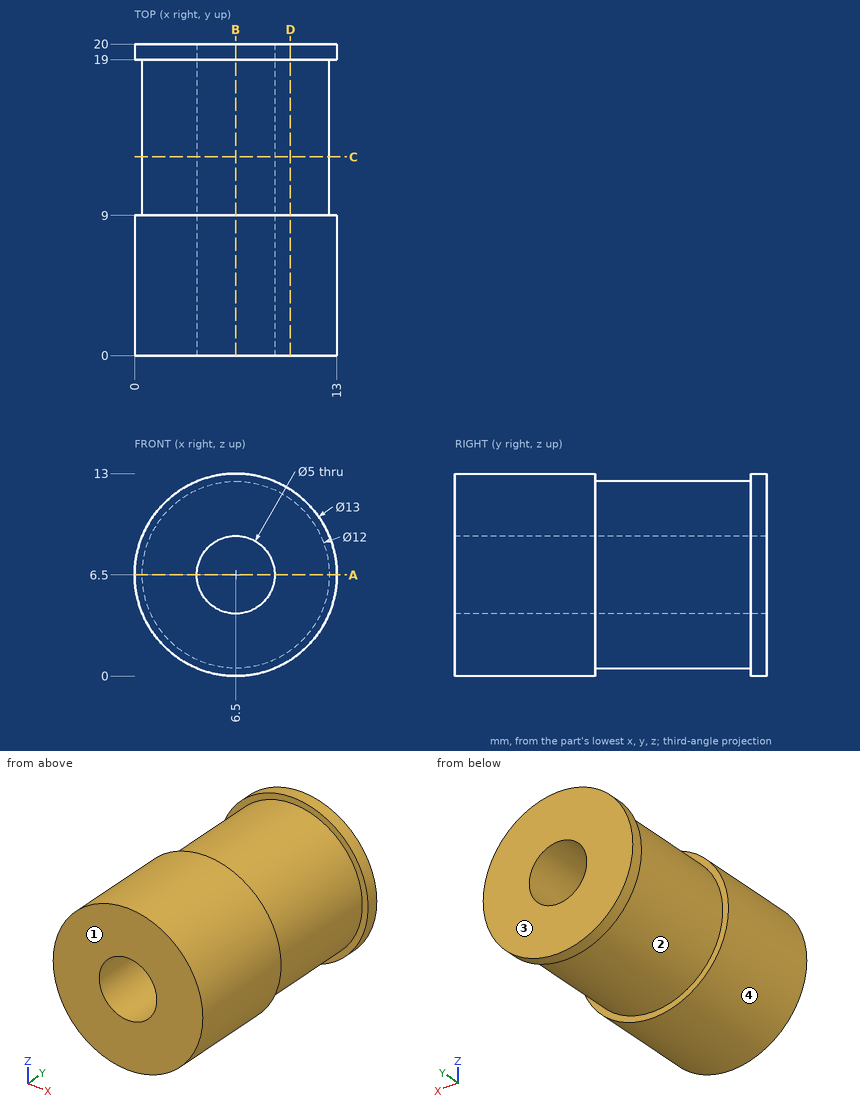
Here's the drawing with two shaded views (mm, measured from the low corner). I have some questions. Round coordinates to 2 decimals unless told otherwise and drop trailing zeros. Order: outer loops, then holes, each group sorted by start corner. A loop starts at its lowest first (then second) coordinate and runs counter-clockwise, first axis right, second up. Notation, with made-up numbers: M 22.5,-22.5 L 81.5,-22.5 A29 ccw 81.5,15.5 Z; hole C 19.25,51 d7. An arc over 180 degrees is marked long. Answer in a Markdown table with one row per item.
Item 1: Imagine slicing it at D-D, the plane x = 10. Write out the boundary of the cut face in (y, z).
A:
| item | result |
|---|---|
| outline | M 0,1.02 L 9,1.02 L 9,1.63 L 19,1.63 L 19,1.02 L 20,1.02 L 20,11.98 L 19,11.98 L 19,11.37 L 9,11.37 L 9,11.98 L 0,11.98 Z |
Item 2: Thinking about a two-plate mould opening in Y: for the marked faces 1, 2, 3 and 4, which applies, +Y half, -Y half, draft (parallel to the pull), parting line (faces both ways), or undercut?
A:
| item | result |
|---|---|
| face 1 | -Y half |
| face 2 | undercut |
| face 3 | +Y half |
| face 4 | draft |
Item 3: I'm going to push flat-ended pins straight in: pin 1 (5 mm diameter, centred on x = 10, y = 18, fed in from -Z); pin 2 (2 mm diameter, centred on y = 7, z = 10.5, fed in from -X); pin 3 (1 mm diameter, centred on y = 10, z = 5, fed in from +X). Where does each tip first touch, or does it pass through?
A:
| item | result |
|---|---|
| pin 1 | stops at z = 0.11 |
| pin 2 | stops at x = 0.73 |
| pin 3 | stops at x = 12.42 |
Item 4: Imagine slicing it at C-C, the plane y = 12.75. Write out the boundary of the cut face in (x, z), and give its area (3 significant figures).
A:
| item | result |
|---|---|
| outline | C 6.5,6.5 d12; hole C 6.5,6.5 d5 |
| area | 93.5 mm2 |
Item 5: If I drill on L1, parallel to X at y = 8.25, z = 6.5; L2, parallel to X at y = 10.5, z = 6.5; L3, parallel to X at y = 1.75, z = 2.5, over which ranges is the centre line in solid material (lowest first)? Write a range as from..to.
A:
| item | result |
|---|---|
| L1 | x = 0..4, 9..13 |
| L2 | x = 0.5..4, 9..12.5 |
| L3 | x = 1.38..11.62 |
Item 6: Imagine slicing it at B-B, the plane x = 6.5. Write out the boundary of the cut face in (y, z), and give its area (3 significant figures).
A:
| item | result |
|---|---|
| outline | M 0,0 L 9,0 L 9,0.5 L 19,0.5 L 19,0 L 20,0 L 20,4 L 0,4 Z; M 0,9 L 20,9 L 20,13 L 19,13 L 19,12.5 L 9,12.5 L 9,13 L 0,13 Z |
| area | 150 mm2 |
Item 7: Imagine slicing it at A-A, the plane z = 6.5. Write out the boundary of the cut face in (x, y), and give its area (3 significant figures).
A:
| item | result |
|---|---|
| outline | M 0,0 L 4,0 L 4,20 L 0,20 L 0,19 L 0.5,19 L 0.5,9 L 0,9 Z; M 9,0 L 13,0 L 13,9 L 12.5,9 L 12.5,19 L 13,19 L 13,20 L 9,20 Z |
| area | 150 mm2 |
